Geometry check sheet. Reference: the model listing, model coordinates, mm. Face numbers are marked on the shaded views. A direction names the side the tool comes from. Give positions to 0.01 mm unless a question says otherwise; leave off trailing zeros. Loops run counter-clockwise (first coordinate to the right, second up) from the corner with the lowest first, then second, coordinate; pieces in that order, holes last. Notation, with made-up numbers: (58, 29.25) -> (70, 29.25) arc R23 ccw to (70, 55.25) -> close; hole circle Ø8 at (-34.75, 58). An arc over 180 degrees is marked (long way). Write item = value, one per line. Start each with the question number.
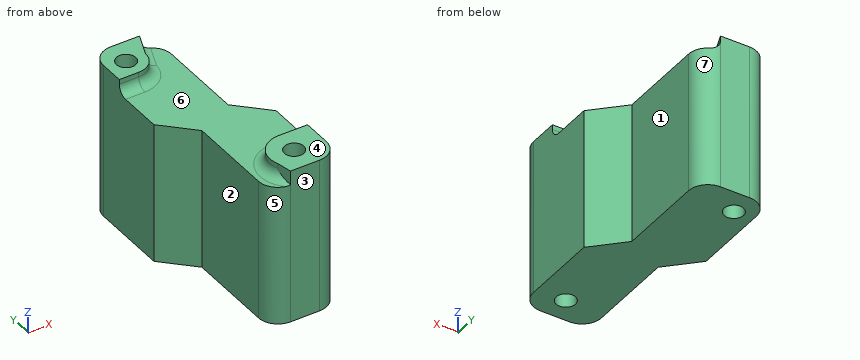
Autodesk Inventor part; units mm, degrees
ref_plane "YZ Plane" through (0, 0, 0) normal (1, 0, 0) x (0, 1, 0)
ref_plane "XZ Plane" through (0, 0, 0) normal (0, 1, 0) x (-1, 0, 0)
ref_plane "XY Plane" through (0, 0, 0) normal (0, 0, 1) x (1, 0, 0)
sketch "Sketch1" plane through (0, 0, 0) normal (0, 0, 1) x (1, 0, 0)
  line L0 (-5, 12) -> (5, 12)
  line L1 (5, 12) -> (5, -12)
  line L2 (5, -12) -> (-5, -12)
  line L3 (-5, -12) -> (-5, 12)
  point P0 (0, 0)
  dimension "d0" = 10
  dimension "d1" = 24
  dimension "d2" = 12
  dimension "d3" = 5
extrude "Extrusion1" add sketch "Sketch1" along normal blind 16
sketch "Sketch2" plane through (0, 0, 16) normal (0, 0, 1) x (1, 0, 0)
  line L0 (-5, -12) -> (5, -12)
  line L1 (5, -12) -> (5, 12)
  circle A0 centre (2, -9.5) radius 1
  point P0 (0, 0)
  point P1 (-2.9408, 9.031)
  dimension "d6" = 2.5
  dimension "d7" = 3
  dimension "d8" = 2
extrude "Extrusion2" cut sketch "Sketch2" against normal blind 16
sketch "Sketch3" plane through (0, 0, 16) normal (0, 0, 1) x (1, 0, 0)
  circle A0 centre (2, -9.5) radius 1
  circle A1 centre (-3, 9.5) radius 1
  point P0 (0, 0)
  point P1 (23.854, -2.3999)
  dimension "d11" = 5
  dimension "d12" = 19
  dimension "d13" = 2
extrude "Extrusion3" cut sketch "Sketch3" against normal blind 16 contours A1
sketch "Sketch4" plane through (0, 0, 16) normal (0, 0, 1) x (1, 0, 0)
  line L0 (-5, 12) -> (-5, -12)
  line L1 (-5, -12) -> (-2, -12)
  line L2 (-2, -12) -> (-2, 2)
  line L3 (-2, 2) -> (-5, 2)
  line L4 (-5, 2) -> (-5, -12)
  line L5 (5, -12) -> (5, 12)
  line L6 (5, 12) -> (2, 12)
  line L7 (2, 12) -> (2, -2)
  line L8 (2, -2) -> (5, -2)
  line L9 (5, -2) -> (5, 12)
  point P0 (0, 0)
  dimension "d16" = 3
  dimension "d17" = 3
  dimension "d18" = 14
  dimension "d19" = 14
extrude "Extrusion4" cut sketch "Sketch4" against normal blind 16
chamfer "Chamfer1" distance 3 angle 45 2 edges at (-2, 2, 8) (2, -2, 8)
fillet "Fillet1" radius 2 4 edges at (-5, 12, 8) (2, 12, 8) (5, -12, 8) (-2, -12, 8)
sketch "Sketch5" plane through (0, 0, 16) normal (0, 0, 1) x (1, 0, 0)
  circle A0 centre (-3, 9.5) radius 1
  circle A1 centre (-3, 9.5) radius 2
  line L0 (-5, 10) -> (-5, 2)
  circle A2 centre (2, -9.5) radius 1
  circle A3 centre (2, -9.5) radius 2.5
  line L1 (0, -12) -> (3, -12)
  line L2 (-5, 12) -> (5, 12)
  line L3 (5, 12) -> (5, -12)
  line L4 (5, -12) -> (-5, -12)
  line L5 (-5, -12) -> (-5, 12)
  line L6 (0, 12) -> (-3, 12)
  line L7 (5, -10) -> (5, -2)
  line L8 (-2, -1) -> (-2, -10)
  line L9 (2, -7) -> (5, -7)
  line L10 (-3, 7.5) -> (-5, 7.5)
  arc A4 (2, 10) -> (0, 12) centre (0, 10) ccw
  line L11 (-1, 9.5) -> (0, 12)
  line L12 (0, 12) -> (-5, 12)
  line L13 (-0.5, -9.5) -> (0, -12)
  point P0 (0, 0)
  point P1 (-0.3077, -10.4615)
extrude "Extrusion5" cut sketch "Sketch5" against normal blind 1.5 contours A1 L11 L2 L3 L9 A3 L13 L4 L5 L0 L10
fillet "Fillet2" radius 1 5 edges at (-0.5, 10.75, 14.5) (-4, 7.5, 14.5) (-1.5858, 8.0858, 14.5) (-0.0801, -8.1132, 14.5) (3.5, -7, 14.5)
properties part number "bridge_structure_C"
1) Draft check along Y on the marked faces 4, 5, 6 and 7. Enter one of: released by +Y, released by -Y, zero draft, split by the parting line, or undercut.
2) Section check D-D (x = 4). Enter the section's corners in (y, z), plus the area to 3 significant figures.
3) Tool access check on the marked faces 1, 2 and 3. Record the directions out of +Z, -Z, +X, -X, +Y, -Y that give a thin tool (end or side, any length) a straight path to the whole face; none if there is none.
4) Depth check by flat-ended pin: pin 1 Ø5 at (x, y) = (3, 0) entering from +Z; pin 2 Ø1 at (y, z) = (0, 5) entering from +X; pin 3 Ø1.5 at (y, z) = (-1, 2.5) entering from -X; pin 4 Ø2.5 at (x, y) = (-3, 9.5) entering from +Z. Enter the tip coordinate at first touch or a pass-through.
5) Section check C-C (x = -3.75). Enter the section's corners in (y, z).
6) Section check A-A (z = 9). Give the number of separate pieces and of enclosed holes in the cut face, plus the area to 3 significant figures.
7) Thickness scan on line 1 (Y direction, x = -3, z = 6.5); line 2 (Z direction, x = -0.75, y = 6); line 3 (Y direction, x = -0.5, z = 12.5). Record the ranges inside material, lowest first.
8) Section check B-B (y = -9.5). Enter the section's corners in (x, z), plus the area to 3 significant figures.
Check result:
q1.face_4 = zero draft
q1.face_5 = released by -Y
q1.face_6 = undercut
q1.face_7 = released by +Y
q2.outline = (-11.73, 0) -> (-1, 0) -> (-1, 14.5) -> (-6, 14.5) arc R1 cw to (-7, 15.5) -> (-7, 16) -> (-11.73, 16) -> close
q2.area = 163 mm2
q3.face_1 = +Z, -Z, +X, +Y
q3.face_2 = +Z, -Z, -X, -Y
q3.face_3 = +Z, -Z, +X, -X, -Y
q4.pin_1 = 14.5
q4.pin_2 = 3.5
q4.pin_3 = -2.75
q4.pin_4 = 16
q5.outline = (0.75, 0) -> (8.84, 0) -> (8.84, 16) -> (7.5, 16) -> (7.5, 15.5) arc R1 cw to (6.5, 14.5) -> (0.75, 14.5) -> close; (10.16, 0) -> (11.85, 0) -> (11.85, 16) -> (10.16, 16) -> close
q6.separate_pieces = 1
q6.enclosed_holes = 2
q6.area = 155 mm2
q7.line_1 = 0 to 8.5, 10.5 to 12
q7.line_2 = 0 to 14.5
q7.line_3 = -11.94 to 12
q8.outline = (-2, 0) -> (1, 0) -> (1, 16) -> (-0.5, 16) -> (-0.5, 15.5) arc R1 cw to (-1.5, 14.5) -> (-2, 14.5) -> close; (3, 0) -> (5, 0) -> (5, 16) -> (3, 16) -> close
q8.area = 78.0 mm2
